from build123d import *

# Parameters (mm, degrees)
F0_W     = 6
F0_H     = 44.3611480296
F1_DEPTH = 190
F3_DEPTH = 500
F4_W     = 65
F4_H     = 50
F5_DEPTH = 500
F6_R     = 2
F7_R     = 5


with BuildPart() as f1:
    # F0 (on Front) → F1 (new body, symmetric)
    with BuildSketch(Plane.XZ):
        Polygon((169.1134991124, 0), (0, 0), (-169.1134991124, 0), (-175.1134991124, 0), (-175.1134991124, -56), (-169.1134991124, -56), (-169.1134991124, -6), (0, -6), (169.1134991124, -6), (169.1134991124, -56), (175.1134991124, -56), (175.1134991124, 0), (175.1134991124, 44.3611480296), (169.1134991124, 44.3611480296), align=None)
        with Locations((-172.1134991124, 22.1805740148)):
            Rectangle(F0_W, F0_H)
    extrude(amount=F1_DEPTH, both=True)

    # F2 (on face) → F3 (cut)
    with BuildSketch(Plane.YZ.offset(175.1134991124)):
        Polygon((-125, 0), (0, 0), (125, 0), (125, 44.3611480296), (-125, 44.3611480296), align=None)
    extrude(amount=-F3_DEPTH, mode=Mode.SUBTRACT)

    # F4 (on face) → F5 (cut)
    with BuildSketch(Plane(origin=(-175.1134991124, 0, 0), x_dir=(0, -1, 0), z_dir=(-1, 0, 0))):
        with Locations((-157.5, -31)):
            Rectangle(F4_W, F4_H)
        with Locations((157.5, -31)):
            Rectangle(F4_W, F4_H)
    extrude(amount=-F5_DEPTH, mode=Mode.SUBTRACT)

    # F6
    f6_edges = [f1.edges().sort_by_distance(p)[0] for p in [
        (169.113499, 157.5, 0),
        (169.113499, -157.5, 0),
        (175.113499, 0, 0),
        (169.113499, 0, -6),
        (175.113499, -157.5, -6),
        (175.113499, 157.5, -6),
        (-169.113499, 157.5, 0),
        (-169.113499, -157.5, 0),
        (-175.113499, 0, 0),
        (-175.113499, -157.5, -6),
        (-169.113499, 0, -6),
        (-175.113499, 157.5, -6),
    ]]
    fillet(f6_edges, radius=F6_R)

    # F7
    f7_edges = [f1.edges().sort_by_distance(p)[0] for p in [
        (172.113499, -190, 44.361148),
        (172.113499, -125, 44.361148),
        (-172.113499, -190, 44.361148),
        (-172.113499, -125, 44.361148),
        (-172.113499, 190, 44.361148),
        (-172.113499, 125, 44.361148),
        (172.113499, 125, 44.361148),
        (172.113499, 190, 44.361148),
        (172.113499, 125, -56),
        (172.113499, -125, -56),
        (-172.113499, -125, -56),
        (-172.113499, 125, -56),
    ]]
    fillet(f7_edges, radius=F7_R)


solid = f1.part
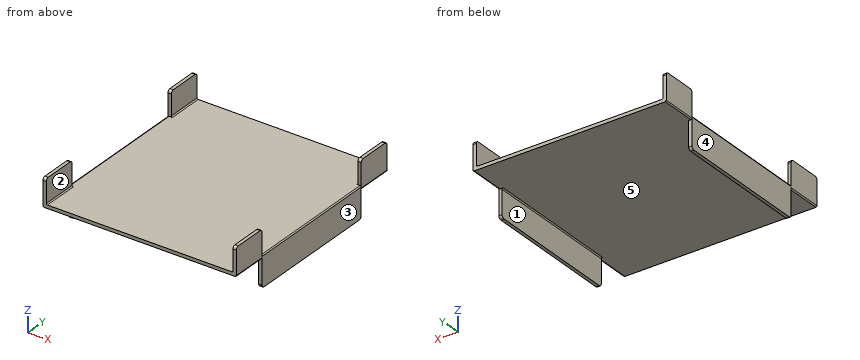
Design review of the part built by this model. Coordinates are the model's own, in mm. Face numbers are marked on the shaded views. A direction names the side the tool comes from. Give positions to 0.01 mm unless a question says otherwise; leave off trailing zeros. Loops run counter-clockwise (first coordinate to the right, second up) from the corner with the lowest first, then second, coordinate; pieces in that order, holes last. Notation, with made-up numbers: M 13,27.25 L 42,27.25 A16 cw 42,35.25 Z; hole C 73,-0.5 d9. An arc over 180 degrees is marked long. Write item = value, one per line.
Q1. To check wall thickness, follow line 1 (X direction, y = -115, z = -33); line 2 (Z direction, x = 23, y = -13). State the ranges of each line that lie inside material, in increasing order. Write a range as [from, to].
Output values:
line_1 = [-175.11, -169.11], [169.11, 175.11]
line_2 = [-6, 0]
Q2. We need section C-C (y = 150). Give the boundary of the cut face in (x, z), plus the area to 3 significant figures.
Output values:
outline = M -175.11,-4 A2 ccw -173.11,-6 L 173.11,-6 A2 ccw 175.11,-4 L 175.11,44.36 L 169.11,44.36 L 169.11,2 A2 cw 167.11,0 L -167.11,0 A2 cw -169.11,2 L -169.11,44.36 L -175.11,44.36 Z
area = 2,630 mm^2
Q3. We need section B-B (z = 20). Give the boundary of the cut face in (x, y).
Output values:
outline = M -175.11,-190 L -169.11,-190 L -169.11,-125 L -175.11,-125 Z; M -175.11,125 L -169.11,125 L -169.11,190 L -175.11,190 Z; M 169.11,-190 L 175.11,-190 L 175.11,-125 L 169.11,-125 Z; M 169.11,125 L 175.11,125 L 175.11,190 L 169.11,190 Z
Q4. For the marked faces 1 and 2, list the 3-axis set-ups (+Z, -Z, +X, -X, +Y, -Y) from which the entire face can be reached by the end or side of a thin tool; tool diameter is ignored.
Output values:
face_1 = -Z, +Y, -Y
face_2 = +Z, +Y, -Y
Q5. Draft analysis for pull direction X (two halves, no side actions). For the marked faces 3, 4 and 5, state which applies: +X half, -X half, draft (parallel to the pull), parting line (faces both ways), or undercut.
Output values:
face_3 = +X half
face_4 = -X half
face_5 = undercut
Q6. Insertion check: pin 1 (3 mm diameter, centred on x = 67.5, y = 68, fed in from +Z); pin 2 (4 mm diameter, centred on x = -171, z = -32.5, fed in from -Y); pin 3 (6 mm diameter, centred on x = 107.5, y = -50, fed in from -Z). Each pin has a flat end and moves straight along its axis. Give the tip position at first contact, or say it passes through.
Output values:
pin_1 = 0
pin_2 = -125
pin_3 = -6
Q7. We need section A-A (z = -31). Give the boundary of the cut face in (x, y), plus the area to 3 significant figures.
Output values:
outline = M -175.11,-125 L -169.11,-125 L -169.11,125 L -175.11,125 Z; M 169.11,-125 L 175.11,-125 L 175.11,125 L 169.11,125 Z
area = 3,000 mm^2
Q8. We need section D-D (x = 112). Give the boundary of the cut face in (y, z), plus the area to 3 significant figures.
Output values:
outline = M -190,-6 L 190,-6 L 190,0 L -190,0 Z
area = 2,280 mm^2
